Geometry check sheet. Reference: drawing and pictorial views, mm from the part's lowest x, y, z. A direction names the side the tool comes from. Round coordinates to 2 decimals unless told otherwise and drop trailing zeros. Order: outer loops, then holes, each group sorted by start corner. A loop starts at its lowest first (then second) coordinate and runs counter-clockwise, first axis right, second up.
Q1. Mould release check, pull along Y, two halves, no side actions. Record for the marked faces 4, 5, 6 and 7: +Y half, -Y half, draft (parallel to the pull), parting line (faces both ways), or undercut.
Q2. Cross-section at A-A on x = 107.95. Record the cut outline in (y, z).
Q3. Cross-section at B-B on y = 23. Give the number of separate pieces and of enclosed holes in the cut face, then the cut area to 3 significant figures.
Q4. Set-up check for the marked faces 1, 2 and 3: record each of +Z, -Z, +X, -X, +Y, -Y from which the full face is reachable in a straight line by a thin tool's end or side.
Q5. Scan lines: probe 1 along Y at (x, z) = (107.95, 4.5); probe 2 along Z at (x, y) = (111.5, 30); probe 3 along X at (y, z) = (16.5, 7) (1 decimal). Record each from-to range of solid material in increasing order.
Q6. Depth check by flat-ended pin: P1, Ø2, axis at x = 39.5, y = 5.5, coming from the +Z side; P2, Ø2, axis at x = 33, z = 15, coming from the +Y side; P3, Ø3, axis at y = 18.5, z = 33.5, coming from the -X side; P4, Ø5, axis at y = 10.5, z = 24, coming from the -X side. Enter the tip coordinate at first touch or a pass-through.
Q7. Cross-section at C-C on z = 22. Record the cut outline in (x, y) (1 decimal).
Q8. Cross-section at D-D on z = 4.5. Record the cut outline in (x, y), then the cut area to 3 significant figures.
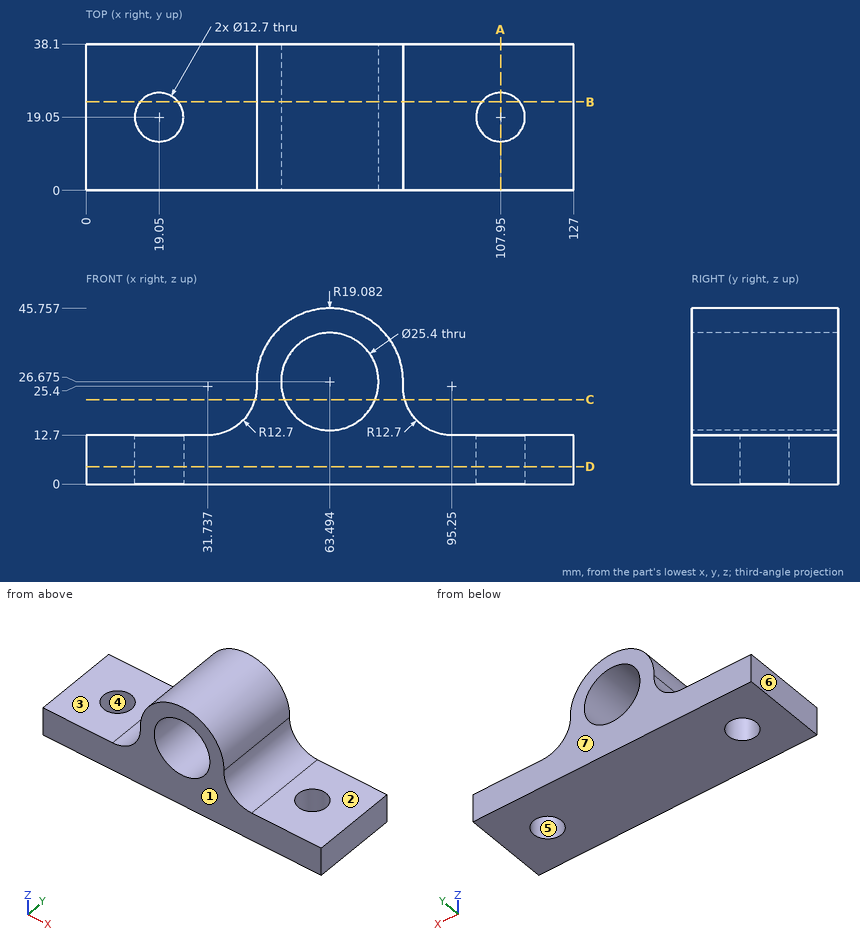
Results found:
1. face 4: undercut
1. face 5: undercut
1. face 6: draft
1. face 7: +Y half
2. outline: (0, 0) - (12.7, 0) - (12.7, 12.7) - (0, 12.7) - close; (25.4, 0) - (38.1, 0) - (38.1, 12.7) - (25.4, 12.7) - close
3. separate pieces: 3
3. enclosed holes: 1
3. area: 2,030 mm2
4. face 1: +Z, -Z, +X, -X, -Y
4. face 2: +Z, +X, +Y, -Y
4. face 3: +Z, -X, +Y, -Y
5. probe 1: y = 0 to 12.7, 25.4 to 38.1
5. probe 2: z = 0 to 12.7
5. probe 3: x = 0 to 13.2, 24.9 to 102.1, 113.8 to 127
6. P1: stops at z = 16.21
6. P2: passes through
6. P3: stops at x = 45.17
6. P4: stops at x = 43.82
7. outline: (44, 0) - (51.7, 0) - (51.7, 38.1) - (44, 38.1) - close; (75.3, 0) - (83, 0) - (83, 38.1) - (75.3, 38.1) - close
8. outline: (0, 0) - (127, 0) - (127, 38.1) - (0, 38.1) - close; hole circle Ø12.7 at (19.05, 19.05); hole circle Ø12.7 at (107.95, 19.05)
8. area: 4,590 mm2
